Check sheet for the modelled part. Datum: model origin and axes. Units: mm. Give positions to 0.01 mm unless a question says otherwise; leave off trailing zeros. Order: outer loops, then holes, each group sorted by start corner. A loop starts at its lowest first (then second) coordinate and runs counter-clockwise, first axis right, second up.
```python
from build123d import *

# Parameters (mm, degrees)
SKETCH1_W           = 99.999999898
SKETCH1_H           = 149.999999974
BOSS_EXTRUDE1_DEPTH = 3
SKETCH2_R           = 1.500000048
SKETCH2_R_2         = 1.5
CUT_EXTRUDE1_DEPTH  = 3


with BuildPart() as part:
    # Sketch1 → Boss-Extrude1 (new body)
    with BuildSketch(Plane(origin=(0, 0, 0), x_dir=(1, 0, 0), z_dir=(0, 1, 0))):
        Rectangle(SKETCH1_W, SKETCH1_H)
    extrude(amount=BOSS_EXTRUDE1_DEPTH)

    # Sketch2 → Cut-Extrude1 (cut)
    with BuildSketch(Plane(origin=(0, 3, 0), x_dir=(1, 0, 0), z_dir=(0, 1, 0))):
        with Locations(Location((-44.919999949, 69.919999987, 0), (0, 0, 270))):
            Circle(SKETCH2_R)
        with Locations(Location((44.919999949, 69.919999987, 0), (0, 0, 270))):
            Circle(SKETCH2_R_2)
        with Locations(Location((-44.919999949, -69.919999987, 0), (0, 0, 270))):
            Circle(SKETCH2_R_2)
        with Locations(Location((44.919999949, -69.919999987, 0), (0, 0, 270))):
            Circle(SKETCH2_R_2)
    extrude(amount=-CUT_EXTRUDE1_DEPTH, mode=Mode.SUBTRACT)


solid = part.part
```
Q1. Sectioned sample at A-A, the plane z = -69.92. Record the cut outline in (x, y), plus the area to 3 significant figures.
Q2. Material ranges on line 1 (Z direction, x = 44.92, y = 2.3); line 2 (X direction, y = 2.1, z = -69.92), recorded low to high.
Q3. Sectioned sample at B-B, the plane x = 44.92. Record the cut outline in (y, z), plus the area to 3 significant figures.
Q4. Go/stop test with flat-tipped pins: P1, Ø3.5, axis at x = 44.92, z = -69.92, coming from the +Y side; P2, Ø1.8, axis at x = -44.92, z = 69.92, coming from the +Y side. Record where each tip stops, or that it passes through.
Q5. Draft check along X on faces 1 (the flat face through (-1, 0, -1)), 2 (the flat face through (50, 1, 1)), 3 (the cylindrical face through (-46.25, 1.52, 70.61)), 4 (the cylindrical face through (43.59, 1.52, 70.61)). Enter one of: pulls with the +X half, pulls with the -X half, needs draft (parallel to the pull), parting line crosses it, or undercut.
Filled in:
1. outline: (-50, 0) - (-46.42, 0) - (-46.42, 3) - (-50, 3) - close; (-43.42, 0) - (43.42, 0) - (43.42, 3) - (-43.42, 3) - close; (46.42, 0) - (50, 0) - (50, 3) - (46.42, 3) - close
1. area: 282 mm2
2. line 1: z = -75 to -71.42, -68.42 to 68.42, 71.42 to 75
2. line 2: x = -50 to -46.42, -43.42 to 43.42, 46.42 to 50
3. outline: (0, -75) - (3, -75) - (3, -71.42) - (0, -71.42) - close; (0, -68.42) - (3, -68.42) - (3, 68.42) - (0, 68.42) - close; (0, 71.42) - (3, 71.42) - (3, 75) - (0, 75) - close
3. area: 432 mm2
4. P1: stops at y = 3
4. P2: passes through
5. face 1: needs draft
5. face 2: pulls with the +X half
5. face 3: undercut
5. face 4: undercut
